Autodesk Inventor part; units mm, degrees
ref_plane "YZ Plane" through (0, 0, 0) normal (1, 0, 0) x (0, 1, 0)
ref_plane "XZ Plane" through (0, 0, 0) normal (0, 1, 0) x (-1, 0, 0)
ref_plane "XY Plane" through (0, 0, 0) normal (0, 0, 1) x (1, 0, 0)
sketch "Sketch1" plane through (0, 0, 0) normal (0, 0, 1) x (1, 0, 0)
  line L0 (0, 0) -> (120, 0)
  line L1 (120, 0) -> (120, 100)
  line L2 (120, 100) -> (0, 100)
  line L3 (0, 100) -> (0, 0)
  dimension "d0" = 120
  dimension "d1" = 100
extrude "Extrusion1" add sketch "Sketch1" along normal blind 10
sketch "Sketch2" plane through (0, 0, 10) normal (0, 0, 1) x (1, 0, 0)
  line L0 (15, 19) -> (105, 19) construction
  line L1 (105, 19) -> (105, 81) construction
  line L2 (105, 81) -> (15, 81) construction
  line L3 (15, 81) -> (15, 19) construction
  circle A0 centre (60, 50) radius 8 construction
  line L4 (15, 19) -> (105, 81) construction
  line L5 (105, 19) -> (15, 81) construction
  point P0 (0, 0)
  dimension "d5" = 90
  dimension "d6" = 62
hole "Hole1" at (15, 81, 10) at (105, 81, 10) at (105, 19, 10) at (15, 19, 10) direction (0, 0, -1) diameter 8 end through all
chamfer "Chamfer1" distance 3 angle 45 1 edges at (15, 85, 10)
chamfer "Chamfer2" distance 3 angle 45 3 edges at (105, 85, 10) (105, 23, 10) (15, 23, 10)
sketch "Sketch3" plane through (0, 0, 0) normal (0, 0, -1) x (-1, 0, 0)
  circle A0 centre (-60, 50) radius 8 construction
  circle A1 centre (-60, 50) radius 27 construction
  point P0 (0, 0)
  point P1 (-60, 77)
  point P2 (-87, 50)
  point P3 (-60, 23)
  point P4 (-33, 50)
  dimension "d20" = 54
  dimension "d23" = 360
hole "Hole2" at (60, 77, 0) at (87, 50, 0) at (60, 23, 0) at (33, 50, 0) direction (0, 0, 1) diameter 3 end through all
chamfer "Chamfer3" distance 2 angle 45 4 edges at (60, 75.5, 0) (33, 48.5, 0) (60, 21.5, 0) (87, 48.5, 0)
properties part number "mounting_plate" material "Aluminum 6061"
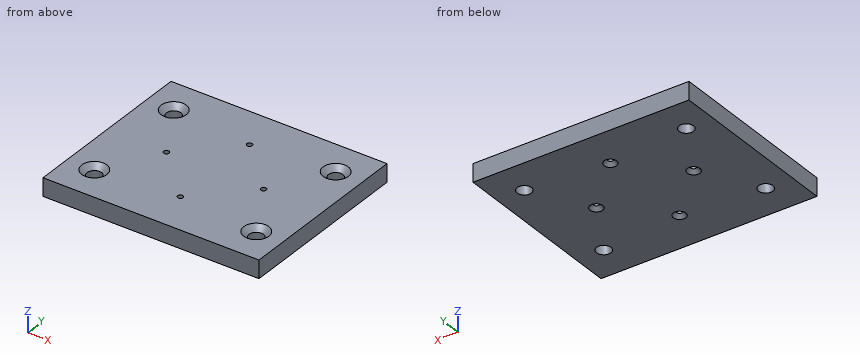
Could you check a few things on this model? Use its own coordinates, in mm. Give positions to 0.01 mm unless a question says otherwise; leave off trailing zeros. Write each loop counter-clockwise with the first axis right and the second up, starting at its lowest first coordinate (ties: lowest second). Pieces come first, ordered by that corner, then holes. Notation, with made-up numbers: (-39, 8.25) -> (-4, 8.25) arc R16 cw to (-4, 17.25) -> close; hole circle Ø2 at (-2.5, 32.25). An arc over 180 degrees is marked (long way). Answer as a JSON object with one key per item and string values.
Q1. Suppose I cut it at B-B on y = 50. Write out the boundary of the cut face in (x, z).
Taken from the geometry:
{"outline": "(0, 0) -> (29.5, 0) -> (31.5, 2) -> (31.5, 10) -> (0, 10) -> close; (34.5, 2) -> (36.5, 0) -> (83.5, 0) -> (85.5, 2) -> (85.5, 10) -> (34.5, 10) -> close; (88.5, 2) -> (90.5, 0) -> (120, 0) -> (120, 10) -> (88.5, 10) -> close"}
Q2. Suppose I cut it at A-A on x = 87. Write out the boundary of the cut face in (y, z).
Taken from the geometry:
{"outline": "(0, 0) -> (46.5, 0) -> (48.5, 2) -> (48.5, 10) -> (0, 10) -> close; (51.5, 2) -> (53.5, 0) -> (100, 0) -> (100, 10) -> (51.5, 10) -> close"}
Q3. Suppose I cut it at D-D on x = 60. Write out the boundary of the cut face in (y, z), then the cut area to 3 significant figures.
Taken from the geometry:
{"outline": "(0, 0) -> (19.5, 0) -> (21.5, 2) -> (21.5, 10) -> (0, 10) -> close; (24.5, 2) -> (26.5, 0) -> (73.5, 0) -> (75.5, 2) -> (75.5, 10) -> (24.5, 10) -> close; (78.5, 2) -> (80.5, 0) -> (100, 0) -> (100, 10) -> (78.5, 10) -> close", "area": "932 mm²"}
Q4. Please list where these lines run through material, in increasing order: L1, parallel to X at y = 50, z = 8.5; L2, parallel to Y at x = 105, z = 1.5; L3, parallel to X at y = 19, z = 4.25.
Taken from the geometry:
{"L1": "x = 0 to 31.5, 34.5 to 85.5, 88.5 to 120", "L2": "y = 0 to 15, 23 to 77, 85 to 100", "L3": "x = 0 to 11, 19 to 101, 109 to 120"}
Q5. Will this pin go through, and if not, where does the flat tip stop? pin 1 Ø3.5 at (x, y) = (60, 23) entering from -Z.
Taken from the geometry:
{"pin 1": "stops at z = 1.75"}
Q6. Suppose I cut it at C-C on z = 5.5. Count the separate pieces of the cut face and the enclosed holes in it, then the cut area to 3 significant figures.
Taken from the geometry:
{"separate pieces": "1", "enclosed holes": "8", "area": "11,800 mm²"}
